The model under review builds one solid part; all positions refer to its coordinate system, in mm. A direction names the side the tool comes from. Round coordinates to 2 decimals unless told otherwise and drop trailing zeros. Loops run counter-clockwise (first coordinate to the right, second up) from the corner with the lowest first, then second, coordinate; pieces in that order, holes last. Notation, with made-up numbers: M 49,56 L 78,56 A26 ccw 78,86 Z; hole C 63.25,-24 d5. An arc over 180 degrees is marked long. Answer in a Markdown table with one row per item. Add a question column.
from build123d import *

# Parameters (mm, degrees)
SKETCH11_R                          = 3.65
BOSCHREXROTH_BOSCH_30X30_V2_1_DEPTH = 406.4


with BuildPart() as part:
    # Sketch11 → Boschrexroth BOSCH_30X30_V2(1) (new body)
    with BuildSketch(Plane.XY.offset(-203.2)):
        with BuildLine():
            Line((0, 5.8), (-4.03, 5.8))
            Line((-4.03, 5.8), (-8.25, 10.02))
            Line((-8.25, 10.02), (-8.25, 12.8))
            Line((-8.25, 12.8), (-4.1, 12.8))
            Line((-4.1, 12.8), (-4.1, 13.9))
            Line((-4.1, 13.9), (-5.1, 13.9))
            Line((-5.1, 13.9), (-5.1, 15))
            Line((-5.1, 15), (-12.5, 15))
            ThreePointArc((-12.5, 15), (-14.267766953, 14.267766953), (-15, 12.5))
            Line((-15, 12.5), (-15, 5.1))
            Line((-15, 5.1), (-13.9, 5.1))
            Line((-13.9, 5.1), (-13.9, 4.1))
            Line((-13.9, 4.1), (-12.8, 4.1))
            Line((-12.8, 4.1), (-12.8, 8.25))
            Line((-12.8, 8.25), (-10.02, 8.25))
            Line((-10.02, 8.25), (-5.8, 4.03))
            Line((-5.8, 4.03), (-5.8, 0))
            Line((-5.8, 0), (-5.8, -4.03))
            Line((-5.8, -4.03), (-10.02, -8.25))
            Line((-10.02, -8.25), (-12.8, -8.25))
            Line((-12.8, -8.25), (-12.8, -4.1))
            Line((-12.8, -4.1), (-13.9, -4.1))
            Line((-13.9, -4.1), (-13.9, -5.1))
            Line((-13.9, -5.1), (-15, -5.1))
            Line((-15, -5.1), (-15, -12.5))
            ThreePointArc((-15, -12.5), (-14.267766953, -14.267766953), (-12.5, -15))
            Line((-12.5, -15), (-5.1, -15))
            Line((-5.1, -15), (-5.1, -13.9))
            Line((-5.1, -13.9), (-4.1, -13.9))
            Line((-4.1, -13.9), (-4.1, -12.8))
            Line((-4.1, -12.8), (-8.25, -12.8))
            Line((-8.25, -12.8), (-8.25, -10.02))
            Line((-8.25, -10.02), (-4.03, -5.8))
            Line((-4.03, -5.8), (4.03, -5.8))
            Line((4.03, -5.8), (8.25, -10.02))
            Line((8.25, -10.02), (8.25, -12.8))
            Line((8.25, -12.8), (4.1, -12.8))
            Line((4.1, -12.8), (4.1, -13.9))
            Line((4.1, -13.9), (5.1, -13.9))
            Line((5.1, -13.9), (5.1, -15))
            Line((5.1, -15), (12.5, -15))
            ThreePointArc((12.5, -15), (14.267766953, -14.267766953), (15, -12.5))
            Line((15, -12.5), (15, -5.1))
            Line((15, -5.1), (13.9, -5.1))
            Line((13.9, -5.1), (13.9, -4.1))
            Line((13.9, -4.1), (12.8, -4.1))
            Line((12.8, -4.1), (12.8, -8.25))
            Line((12.8, -8.25), (10.02, -8.25))
            Line((10.02, -8.25), (5.8, -4.03))
            Line((5.8, -4.03), (5.8, 0))
            Line((5.8, 0), (5.8, 4.03))
            Line((5.8, 4.03), (10.02, 8.25))
            Line((10.02, 8.25), (12.8, 8.25))
            Line((12.8, 8.25), (12.8, 4.1))
            Line((12.8, 4.1), (13.9, 4.1))
            Line((13.9, 4.1), (13.9, 5.1))
            Line((13.9, 5.1), (15, 5.1))
            Line((15, 5.1), (15, 12.5))
            ThreePointArc((15, 12.5), (14.267766953, 14.267766953), (12.5, 15))
            Line((12.5, 15), (5.1, 15))
            Line((5.1, 15), (5.1, 13.9))
            Line((5.1, 13.9), (4.1, 13.9))
            Line((4.1, 13.9), (4.1, 12.8))
            Line((4.1, 12.8), (8.25, 12.8))
            Line((8.25, 12.8), (8.25, 10.02))
            Line((8.25, 10.02), (4.03, 5.8))
            Line((4.03, 5.8), (0, 5.8))
        make_face()
        Circle(SKETCH11_R, mode=Mode.SUBTRACT)
    extrude(amount=BOSCHREXROTH_BOSCH_30X30_V2_1_DEPTH)


solid = part.part
1. Take a section at A-A, the plane y = 0. State the section outline as (x, z) points.
2. Machinability: for faces 4 (the flat face through (5.8, 0, -3)), 5 (the flat face through (0, 5.8, -3)), 6 (the flat face through (-9, 15, -3)), 7 (the flat face through (-5.8, 0, -3)), which of the approach directions +Z, -Z, +X, -X, +Y, -Y give a long, thin tool a straight path to every point of the face, cutting with its end or side? Answer none if there is none.
3. To check wall thickness, follow probe 1 along X at (y, z) = (12.75, -58.5); probe 2 along Y at (x, z) = (0, 35.5); probe 3 along X at (y, z) = (8, -94). State the ranges of each line that lie inside material, in increasing order.
4. Mouldability with a two-part tool opening along X and no side actions: class faces 1 (the flat face through (0, -5.8, -3)), 2 (the flat face through (-4, 4, 203.2)), 3 (the flat face through (-15, -9, -3)) as released by +X, released by -X, zero draft, split by the parting line, or undercut.
5. For pin 1 Ø0.5 at (x, z) = (-13.5, 41) entering from +Y; pin 2 Ø0.9 at (y, z) = (13.5, 53) entering from -X; pin 3 Ø0.9 at (x, z) = (-14.5, -20) entering from +Y, all flat-tipped, find the tip position at first contact; note any pin that passes through.
Check sheet entries:
| question | item | result |
|---|---|---|
| 1 | outline | M -5.8,-203.2 L -3.65,-203.2 L -3.65,203.2 L -5.8,203.2 Z; M 3.65,-203.2 L 5.8,-203.2 L 5.8,203.2 L 3.65,203.2 Z |
| 2 | face 4 | +Z, -Z, +X |
| 2 | face 5 | +Z, -Z, +Y |
| 2 | face 6 | +Z, -Z, +X, -X, +Y |
| 2 | face 7 | +Z, -Z, -X |
| 3 | probe 1 | x = -14.99 to -8.25, 8.25 to 14.99 |
| 3 | probe 2 | y = -5.8 to -3.65, 3.65 to 5.8 |
| 3 | probe 3 | x = -15 to -12.8, -9.77 to -6.23, 6.23 to 9.77, 12.8 to 15 |
| 4 | face 1 | undercut |
| 4 | face 2 | zero draft |
| 4 | face 3 | released by -X |
| 5 | pin 1 | stops at y = 14.88 |
| 5 | pin 2 | stops at x = -14.94 |
| 5 | pin 3 | stops at y = 14.46 |
